Read the model definition and answer for the solid it produces. Units are mm, in the model's axes. A direction names the side the tool comes from. Round coordinates to 2 decimals unless told otherwise and drop trailing zeros. Loops run counter-clockwise (first coordinate to the right, second up) from the corner with the lowest first, then second, coordinate; pieces in that order, holes last. Notation, with made-up numbers: M -25.75,29 L -3.75,29 A24 ccw -3.75,41 Z; hole C 7,5 d1. An arc over 180 degrees is marked long. Write each question's results on one line, items separated by ' | '.
```python
from build123d import *

# Parameters (mm, degrees)
EXTRUDE_1_DEPTH           = 35
HOLE_WIZARD_1_D           = 5.5
HOLE_WIZARD_1_CBORE_D     = 10
HOLE_WIZARD_1_CBORE_DEPTH = 27
SKETCH_6_R                = 5
SKETCH_6_R_2              = 2.75
SKETCH_6_R_3              = 2.861192155
CUT_EXTRUDE_1_DEPTH       = 27
SKETCH_8_R                = 2.75
SKETCH_8_R_2              = 2.861192155
CUT_EXTRUDE_2_DEPTH       = 35
CUT_EXTRUDE_3_DEPTH       = 35
CUT_EXTRUDE_4_DEPTH       = 35


with BuildPart() as part:
    # 草图1 → 凸台-拉伸1 (new body)
    with BuildSketch(Plane.XY):
        Polygon((-30.620689655, 42.965517241), (49.379310345, 42.965517241), (49.379310345, -37.034482759), (29.379310345, -37.034482759), (29.379310345, 22.965517241), (-30.620689655, 22.965517241), align=None)
    extrude(amount=EXTRUDE_1_DEPTH)

    # 孔1 (through all)
    with Locations(Plane(origin=(39.379310345, 32.965517241, 35), x_dir=(1, 0, 0), z_dir=(0, 0, 1))):
        with Locations((0, 0)):
            CounterBoreHole(HOLE_WIZARD_1_D / 2, HOLE_WIZARD_1_CBORE_D / 2, HOLE_WIZARD_1_CBORE_DEPTH)

    # 草图6 → 切除-拉伸1 (cut)
    with BuildSketch(Plane.XY.offset(35)):
        with Locations((14.324422016, 32.985524686)):
            Circle(SKETCH_6_R)
        with Locations((14.324422016, 32.985524686)):
            Circle(SKETCH_6_R_2, mode=Mode.SUBTRACT)
        with Locations((39.242589892, 7.916677332)):
            Circle(SKETCH_6_R)
        with Locations((39.242589892, 7.916677332)):
            Circle(SKETCH_6_R_3, mode=Mode.SUBTRACT)
        with Locations((39.242589892, -17.041261432)):
            Circle(SKETCH_6_R)
        with Locations((39.242589892, -17.041261432)):
            Circle(SKETCH_6_R_2, mode=Mode.SUBTRACT)
        with Locations((-10.641383775, 32.985524686)):
            Circle(SKETCH_6_R)
        with Locations((-10.641383775, 32.985524686)):
            Circle(SKETCH_6_R_2, mode=Mode.SUBTRACT)
    extrude(amount=-CUT_EXTRUDE_1_DEPTH, mode=Mode.SUBTRACT)

    # 草图8 → 切除-拉伸2 (cut)
    with BuildSketch(Plane.XY.offset(35)):
        with Locations((14.324422016, 32.985524686)):
            Circle(SKETCH_8_R)
        with Locations((39.242589892, 7.916677332)):
            Circle(SKETCH_8_R_2)
        with Locations((39.242589892, -17.041261432)):
            Circle(SKETCH_8_R)
        with Locations((-10.641383775, 32.985524686)):
            Circle(SKETCH_8_R)
    extrude(amount=-CUT_EXTRUDE_2_DEPTH, mode=Mode.SUBTRACT)

    # 草图9 → 切除-拉伸3 (cut)
    with BuildSketch(Plane(origin=(49.379310345, 0, 0), x_dir=(0, 0, -1), z_dir=(1, 0, 0))):
        Polygon((-5, -32.034482759), (-30, -7.034482759), (-35, -7.034482759), (-35, -37.034482759), (-5, -37.034482759), align=None)
    extrude(amount=-CUT_EXTRUDE_3_DEPTH, mode=Mode.SUBTRACT)

    # 草图10 → 切除-拉伸4 (cut)
    with BuildSketch(Plane(origin=(0, 42.965517241, 0), x_dir=(1, 0, 0), z_dir=(0, 1, 0))):
        Polygon((-30.620689655, -35), (-0.620689655, -35), (-0.620689655, -30), (-25.620689655, -5), (-30.620689655, -5), align=None)
    extrude(amount=-CUT_EXTRUDE_4_DEPTH, mode=Mode.SUBTRACT)


solid = part.part
```
1. Find section D-D, the plane x = -14.5. Give the vertices of the cut face in (y, z).
Completed:
outline: M 22.97,0 L 42.97,0 L 42.97,16.12 L 36.17,16.12 L 36.17,8 L 29.81,8 L 29.81,16.12 L 22.97,16.12 Z
2. Find section C-C, the plane z = 4. Give the vertices of the cut face in (x, y).
Completed:
outline: M -30.62,22.97 L 29.38,22.97 L 29.38,-37.03 L 49.38,-37.03 L 49.38,42.97 L -30.62,42.97 Z; hole C -10.64,32.99 d5.5; hole C 14.32,32.99 d5.5; hole C 39.24,7.92 d5.72; hole C 39.24,-17.04 d5.5; hole C 39.38,32.97 d5.5
3. Find section B-B, the plane z = 15.5. Give the vertices of the cut face in (x, y), then the cut area to 3 significant figures.
Completed:
outline: M -15.12,22.97 L 29.38,22.97 L 29.38,-21.53 L 37.05,-21.53 A5 cw long 41.44,-21.53 L 49.38,-21.53 L 49.38,42.97 L -15.12,42.97 L -15.12,35.21 A5 cw long -15.12,30.76 Z; hole C 14.32,32.99 d10; hole C 39.24,7.92 d10; hole C 39.38,32.97 d10 | area: 1,790 mm2
4. Find the intervals of material crossed by L1, parallel to X at y = 31.5, z = 18.5; L2, parallel to Y at x = 43, z = 22.5; L3, parallel to Y at x = 40.5, z = 15, in increasing order.
Completed:
L1: x = -5.87 to 9.55, 19.1 to 34.6, 44.16 to 49.38 | L2: y = -13.74 to 4.62, 11.22 to 29.52, 36.41 to 42.97 | L3: y = -22.03 to -21.88, -12.2 to 3.08, 12.76 to 28.09, 37.84 to 42.97
5. Determine the mould class of faces 1 (the face through (13.674, 37.943, 21.689)), 2 (the face through (39.519, -22.487, 14.547)), 3 (the face through (29.379, -1, 13)) for opening direction X: released by +X, released by -X, zero draft, split by the parting line, or undercut.
Completed:
face 1: undercut | face 2: zero draft | face 3: released by -X
6. Find section A-A, the plane y = 25.5. Give the vertices of the cut face in (x, z), then the cut area to 3 significant figures.
Completed:
outline: M -30.62,0 L 49.38,0 L 49.38,35 L -0.62,35 L -0.62,30 L -25.62,5 L -30.62,5 Z | area: 2,210 mm2
7. Which of the six approach directions +Z, -Z, +X, -X, +Y, -Y give full straight-line access (tool end or side, diameter ignored) to faces 4 (the face through (6, 22.966, 13)), 5 (the face through (40, -35, 5)), 6 (the face through (16.5, 30.8, 8)), 7 (the face through (-0.621, 33, 33))?
Completed:
face 4: +Z, -Z, -X, -Y | face 5: +Z, +X, -X, -Y | face 6: +Z | face 7: +Z, -X, +Y, -Y
8. Given P1, Ø4, axis at x = -28.5, y = 34, coming from the +Z side; P2, Ø17.5, axis at y = -14, z = 21.5, coming from the -X side; P3, Ø3, axis at x = 41, y = 34.5, coming from the +Z side, each flat-ended and moving along its own axis, determine where each tip first touches the part or whether it passes through.
Completed:
P1: stops at z = 5 | P2: stops at x = 29.38 | P3: stops at z = 8
